from build123d import *

# Parameters (mm, degrees)
BOSS_EXTRUDE3_DEPTH = 20
SKETCH4_R           = 2.5
CUT_EXTRUDE1_DEPTH  = 20
SKETCH5_R           = 2.5
CUT_EXTRUDE2_DEPTH  = 20
FILLET1_R           = 10
FILLET2_R           = 3


with BuildPart() as part:
    # Sketch3 → Boss-Extrude3 (new body)
    with BuildSketch(Plane(origin=(0, 0, 0), x_dir=(0, 0, -1), z_dir=(1, 0, 0))):
        Polygon((0, 0), (0, 30), (-3, 30), (-3, 3), (-18, 3), (-18, 0), align=None)
    extrude(amount=BOSS_EXTRUDE3_DEPTH)

    # Sketch4 → Cut-Extrude1 (cut)
    with BuildSketch(Plane.XY.offset(3)):
        with Locations((10, 22)):
            Circle(SKETCH4_R)
    extrude(amount=-CUT_EXTRUDE1_DEPTH, mode=Mode.SUBTRACT)

    # Sketch5 → Cut-Extrude2 (cut)
    with BuildSketch(Plane(origin=(0, 3, 0), x_dir=(1, 0, 0), z_dir=(0, 1, 0))):
        with Locations(Location((5, -13, 0), (0, 0, 270))):
            Circle(SKETCH5_R)
        with Locations(Location((15, -13, 0), (0, 0, 270))):
            Circle(SKETCH5_R)
    extrude(amount=-CUT_EXTRUDE2_DEPTH, mode=Mode.SUBTRACT)

    # Fillet1
    fillet1_edges = [part.edges().sort_by_distance(p)[0] for p in [
        (0, 30, 1.5),
        (20, 30, 1.5),
    ]]
    fillet(fillet1_edges, radius=FILLET1_R - 0.0001)  # a hair under: the kernel refuses the full size

    # Fillet2
    fillet2_edges = [part.edges().sort_by_distance(p)[0] for p in [
        (20, 1.5, 18),
        (0, 1.5, 18),
    ]]
    fillet(fillet2_edges, radius=FILLET2_R)


solid = part.part
Could you check a few things on this model? Use its own coordinates, in mm. A direction names the side the tool comes from. Round coordinates to 2 decimals unless told otherwise and drop trailing zeros. Write each loop counter-clockwise with the first axis right and the second up, starting at its lowest first coordinate (ties: lowest second). Pieces come first, ordered by that corner, then holes. Notation, with made-up numbers: (71, 30) - (76, 30) arc R28 ccw to (76, 68) - close; hole circle Ø7 at (18.25, 34.5). An arc over 180 degrees is marked (long way). Use a Markdown table: item, result.
Q1. Please list where these lines run through material, in increasing order: L1, parallel to X at y = 2.4, z = 13; L2, parallel to Y at x = 10, z = 1.7; L3, parallel to Y at x = 14, z = 8.
Output values:
| item | result |
|---|---|
| L1 | 0 to 2.5, 7.5 to 12.5, 17.5 to 20 |
| L2 | 0 to 19.5, 24.5 to 30 |
| L3 | 0 to 3 |
Q2. I want a section at A-A (z = 13). List the corners of the cut face in (x, y) for me.
Output values:
| item | result |
|---|---|
| outline | (0, 0) - (2.5, 0) - (2.5, 3) - (0, 3) - close; (7.5, 0) - (12.5, 0) - (12.5, 3) - (7.5, 3) - close; (17.5, 0) - (20, 0) - (20, 3) - (17.5, 3) - close |
Q3. For faces 1 (the flat face through (10, 17, 3)), 2 (the cylindrical face through (19.14, 1.48, 17.1)), which set-ups out of +Z, -Z, +X, -X, +Y, -Y let a thin tool reach every point of the face, with its end or its side?
Output values:
| item | result |
|---|---|
| face 1 | +Z, +X, -X, +Y |
| face 2 | +Z, +X, +Y, -Y |
Q4. I want a section at B-B (x = 13). List the corners of the cut face in (y, z) for me, plus the area to 3 significant figures.
Output values:
| item | result |
|---|---|
| outline | (0, 0) - (29.54, 0) - (29.54, 3) - (3, 3) - (3, 11.5) - (0, 11.5) - close; (0, 14.5) - (3, 14.5) - (3, 18) - (0, 18) - close |
| area | 125 mm2 |
Q5. Thinking about a two-plate mould opening in X: for faces 3 (the cylindrical face through (13.5, 1.5, 11)), 4 (the flat face through (20, 7.1, 2.5)), 5 (the cylindrical face through (0.86, 1.48, 17.1)), which applies, released by +X, released by -X, zero draft, split by the parting line, or undercut?
Output values:
| item | result |
|---|---|
| face 3 | undercut |
| face 4 | released by +X |
| face 5 | released by -X |
Q6. For pin 1 (4.5 mm diameter, centred on x = 10, y = 22, fed in from +Z); pin 2 (10 mm diameter, centred on x = 5.5, y = 20.5, fed in from +Z); pin 3 (3 mm diameter, centred on x = 17, z = 2.5, fed in from -Y); pin 4 (1 mm diameter, centred on y = 21, z = 3, fed in from -X), each with a flat end and sliding along its axis, tell me the tip position at first contact or that it passes through.
Output values:
| item | result |
|---|---|
| pin 1 | through |
| pin 2 | z = 3 |
| pin 3 | y = 0 |
| pin 4 | x = 0.01 |
Q7. I want a section at D-D (y = 22). List the corners of the cut face in (x, z) for me, plus the area to 3 significant figures.
Output values:
| item | result |
|---|---|
| outline | (0.2, 0) - (7.5, 0) - (7.5, 3) - (0.2, 3) - close; (12.5, 0) - (19.8, 0) - (19.8, 3) - (12.5, 3) - close |
| area | 43.8 mm2 |
